The figure shows three views and two pictorial views of one solid part (mm, origin at its lowest corner). Answer the questions. A direction names the side the tool comes from. Give positions to 0.01 mm unless a question says otherwise; leave off trailing zeros. Loops run counter-clockwise (first coordinate to the right, second up) from the corner with the lowest first, then second, coordinate; pieces in that order, holes last. Notation, with made-up numbers: (-34, -20.5) -> (16, -20.5) arc R10 ccw to (16, -16.5) -> close; hole circle Ø6 at (-4, 57.25). An arc over 180 degrees is marked (long way). One line per item, written item: value. Start each with the question number.
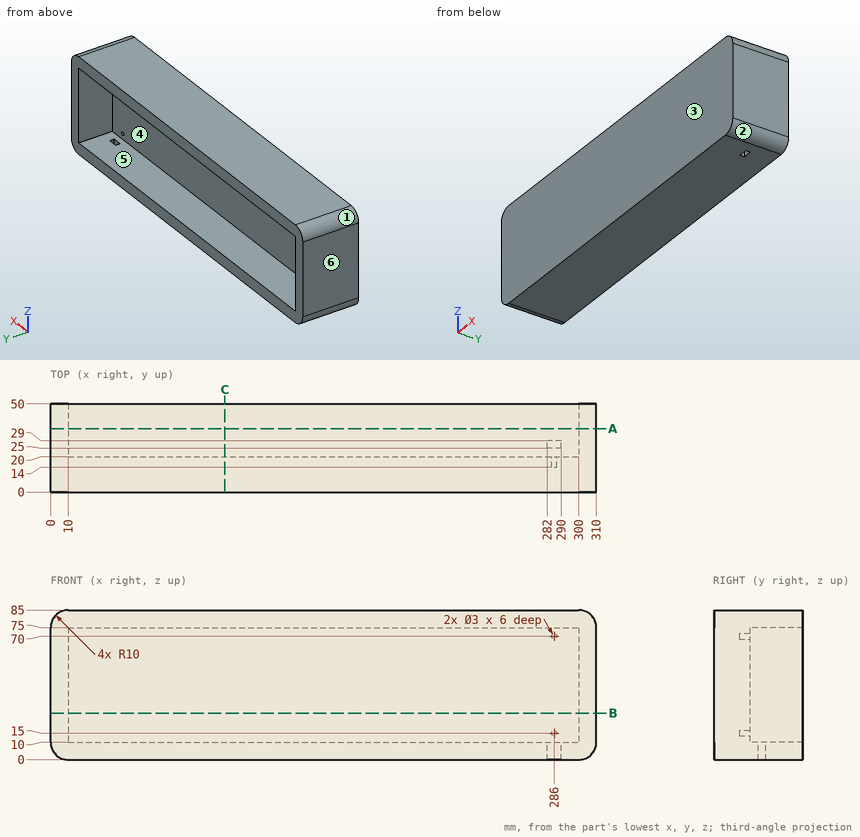
Item 1: Consider L1, parallel to Z at x = 286, y = 16; L2, parallel to Z at x = 183, y = 39; L3, parallel to X at y = 41, z = 20. Determine where each line is inside the solid, lowest interval first. Write a range as [from, to].
Item 2: Flat-ended cylindrical pins translate along their axes: pin 1 (1.5 mm diameter, centred on x = 285.5, z = 15.5, fed in from +Y); pin 2 (4.5 mm diameter, centred on y = 27, z = 7.5, fed in from +X); pin 3 (1.2 mm diameter, centred on y = 27.5, z = 3.5, fed in from -X). Find the tip coordinate at first contact, or state that the pin passes through.
Item 3: Determine the mould class of the marked faces 1, 2, 3 and 4 for opening direction Z: pulls with the +Z half, pulls with the -Z half, needs draft (parallel to the pull), parting line crosses it, or undercut.
Item 4: For the marked faces 5 and 6, determine the directions among +Z, -Z, +X, -X, +Y, -Y from which every point of the face is accessible in a straight line to the end or side of a thin tool.
Item 5: Section C-C, the plane x = 99 is taken. Determine the outline of the cut face in (y, z), plus the area to 3 significant figures.
Item 6: Section B-B, the plane z = 26.5 is taken. Determine the outline of the cut face in (x, y), plus the area to 3 significant figures.
Item 7: Section A-A, the plane y = 36 is taken. Determine the outline of the cut face in (x, z).
Computed values:
1. L1: [0, 13.5], [16.5, 68.5], [71.5, 85]
1. L2: [0, 10], [75, 85]
1. L3: [0, 10], [300, 310]
2. pin 1: y = 14
2. pin 2: x = 310
2. pin 3: x = 1.93
3. face 1: pulls with the +Z half
3. face 2: pulls with the -Z half
3. face 3: needs draft
3. face 4: undercut
4. face 5: +Y
4. face 6: +Z, -Z, -X, +Y, -Y
5. outline: (0, 0) -> (50, 0) -> (50, 10) -> (20, 10) -> (20, 75) -> (50, 75) -> (50, 85) -> (0, 85) -> close
5. area: 2,300 mm²
6. outline: (0, 0) -> (310, 0) -> (310, 50) -> (300, 50) -> (300, 20) -> (10, 20) -> (10, 50) -> (0, 50) -> close
6. area: 6,800 mm²
7. outline: (0, 10) arc R10 ccw to (10, 0) -> (300, 0) arc R10 ccw to (310, 10) -> (310, 75) arc R10 ccw to (300, 85) -> (10, 85) arc R10 ccw to (0, 75) -> close; hole (10, 10) -> (300, 10) -> (300, 75) -> (10, 75) -> close
